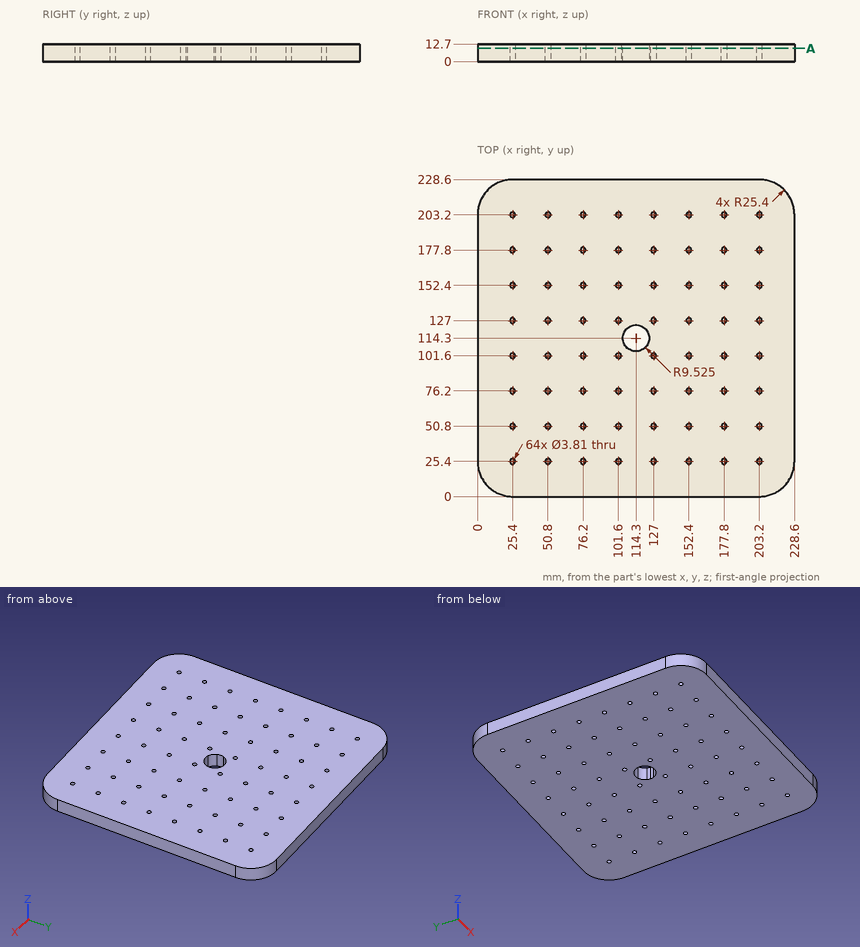
Geometry: see drawing. Coordinates: mm, zero at the bounding-box minimum. Coordinates: 2 decimals unless noted, no trailing zeros. Put each result on its own line as item: value. Start each with the question number.
Q1. Line query: line 1 (Y direction, x = 216.5, z = 6.75). Output: solid intervals per line, ascending.
Q2. Cut plane A-A, the plane z = 9.5. Give the number of separate pieces and of enclosed holes in the cut face, and give its area (3 significant figures).
Q3. Pin query (flat end, axial travel): pin 1 Ø2 at (y, z) = (80.5, 2.5) entering from -X. Return the tip coordinate at first contact, or that it passes through.
Filled sheet:
1. line 1: 3.76 to 224.84
2. separate pieces: 1
2. enclosed holes: 65
2. area: 50,700 mm²
3. pin 1: x = 0
